from build123d import *

# Parameters (mm, degrees)
SKETCH1_W                    = 102
SKETCH1_H                    = 22
EXTRUDE1_DEPTH               = 8
F_4_0_4_DIAMETER_HOLE1_D     = 3.9
F_4_0_4_DIAMETER_HOLE1_DEPTH = 15
SKETCH3_W                    = 30
SKETCH3_H                    = 25
EXTRUDE2_DEPTH               = 8
FILLET1_R                    = 10
F_4_0_4_DIAMETER_HOLE2_D     = 3.9
F_4_0_4_DIAMETER_HOLE2_DEPTH = 15
SKETCH5_W                    = 30
SKETCH5_H                    = 25
EXTRUDE3_DEPTH               = 4


with BuildPart() as part:
    # Sketch1 → Extrude1 (new body)
    with BuildSketch(Plane.XY):
        Rectangle(SKETCH1_W, SKETCH1_H)
    extrude(amount=EXTRUDE1_DEPTH)

    # Ø4.0 (4) Diameter Hole1
    with Locations(Plane(origin=(46.2, 6, 8), x_dir=(1, 0, 0), z_dir=(0, 0, 1))):
        with Locations((0, 0), (0, -12)):
            Hole(F_4_0_4_DIAMETER_HOLE1_D / 2, depth=F_4_0_4_DIAMETER_HOLE1_DEPTH)

    # Sketch3 → Extrude2 (add)
    with BuildSketch(Plane.XY):
        with Locations((-36, 23.5)):
            Rectangle(SKETCH3_W, SKETCH3_H)
    extrude(amount=EXTRUDE2_DEPTH)

    # Fillet1
    fillet1_edges = [part.edges().sort_by_distance(p)[0] for p in [
        (-51, -11, 4),
    ]]
    fillet(fillet1_edges, radius=FILLET1_R)

    # Ø4.0 (4) Diameter Hole2
    with Locations(Plane(origin=(-46, 16, 8), x_dir=(1, 0, 0), z_dir=(0, 0, 1))):
        with Locations((0, 0), (20, 0), (10, 16)):
            Hole(F_4_0_4_DIAMETER_HOLE2_D / 2, depth=F_4_0_4_DIAMETER_HOLE2_DEPTH)

    # Sketch5 → Extrude3 (cut)
    with BuildSketch(Plane.XY.offset(8)):
        with Locations((-36, 23.5)):
            Rectangle(SKETCH5_W, SKETCH5_H)
    extrude(amount=-EXTRUDE3_DEPTH, mode=Mode.SUBTRACT)


solid = part.part
Read the model definition and answer for the solid it produces. Units are mm, in the model's axes. A direction names the side the tool comes from. Round coordinates to 2 decimals unless told otherwise and drop trailing zeros. Loops run counter-clockwise (first coordinate to the right, second up) from the corner with the lowest first, then second, coordinate; pieces in that order, holes last.
Q1. Consider probe 1 along Y at (x, z) = (46.2, 5.25); probe 2 along Y at (x, z) = (-34, 7.25); probe 3 along Y at (x, z) = (-36, 2.1). Determine where each line is inside the solid, lowest interval first.
Q2. Section C-C on z = 2.25 is taken. Write down the section's boundary in (x, y), and give its area (3 significant figures).
Q3. Each of these flat-tipped pins is pushed along its axis until it touches: pin 1 (1 mm diameter, centred on y = -3.5, z = 3.5, fed in from -X); pin 2 (8 mm diameter, centred on x = -22.5, y = 30.5, fed in from +Z); pin 3 (2 mm diameter, centred on x = 35.5, y = -2, fed in from -Z); pin 4 (4.5 mm diameter, centred on y = 24.5, z = 2.5, fed in from +X). Where does it stop, or does it pass through?
Q4. Section D-D on x = 46.2 is taken. Write down the section's boundary in (y, z), and give its area (3 significant figures).
Q5. Section A-A on y = 16 is taken. Write down the section's boundary in (x, z), and give its area (3 significant figures).
Q6. Section B-B on y = 6 is taken. Write down the section's boundary in (x, z), and give its area (3 significant figures).
Q7. Determine the mould class of faces 3 (the face through (48.148, 6.086, 3.944)), 4 (the face through (51, 0, 4)), 5 (the face through (-36, 24, 4)), 6 (the face through (-51, 13, 3)) for opening direction X: released by +X, released by -X, zero draft, split by the parting line, or undercut.
Q8. Which of the six approach directions +Z, -Z, +X, -X, +Y, -Y give full straight-line access (tool end or side, diameter ignored) to faces 1 (the face through (-21, 23, 2)), 2 (the face through (-37.048, 33.644, 1.972))?
Output:
1. probe 1: y = -11 to -7.95, -4.05 to 4.05, 7.95 to 11
1. probe 2: y = -11 to 11
1. probe 3: y = -11 to 30.05, 33.95 to 36
2. outline: (-51, -1) arc R10 ccw to (-41, -11) - (51, -11) - (51, 11) - (-21, 11) - (-21, 36) - (-51, 36) - close; hole circle Ø3.9 at (-46, 16); hole circle Ø3.9 at (-36, 32); hole circle Ø3.9 at (-26, 16); hole circle Ø3.9 at (46.2, -6); hole circle Ø3.9 at (46.2, 6)
2. area: 2,910 mm2
3. pin 1: stops at x = -50.8
3. pin 2: stops at z = 4
3. pin 3: stops at z = 0
3. pin 4: stops at x = -21
4. outline: (-11, 0) - (-7.95, 0) - (-7.95, 8) - (-11, 8) - close; (-4.05, 0) - (4.05, 0) - (4.05, 8) - (-4.05, 8) - close; (7.95, 0) - (11, 0) - (11, 8) - (7.95, 8) - close
4. area: 114 mm2
5. outline: (-51, 0) - (-47.95, 0) - (-47.95, 4) - (-51, 4) - close; (-44.05, 0) - (-27.95, 0) - (-27.95, 4) - (-44.05, 4) - close; (-24.05, 0) - (-21, 0) - (-21, 4) - (-24.05, 4) - close
5. area: 88.8 mm2
6. outline: (-51, 0) - (44.25, 0) - (44.25, 8) - (-51, 8) - close; (48.15, 0) - (51, 0) - (51, 8) - (48.15, 8) - close
6. area: 785 mm2
7. face 3: undercut
7. face 4: released by +X
7. face 5: zero draft
7. face 6: released by -X
8. face 1: +Z, -Z, +X, +Y
8. face 2: +Z, -Z
